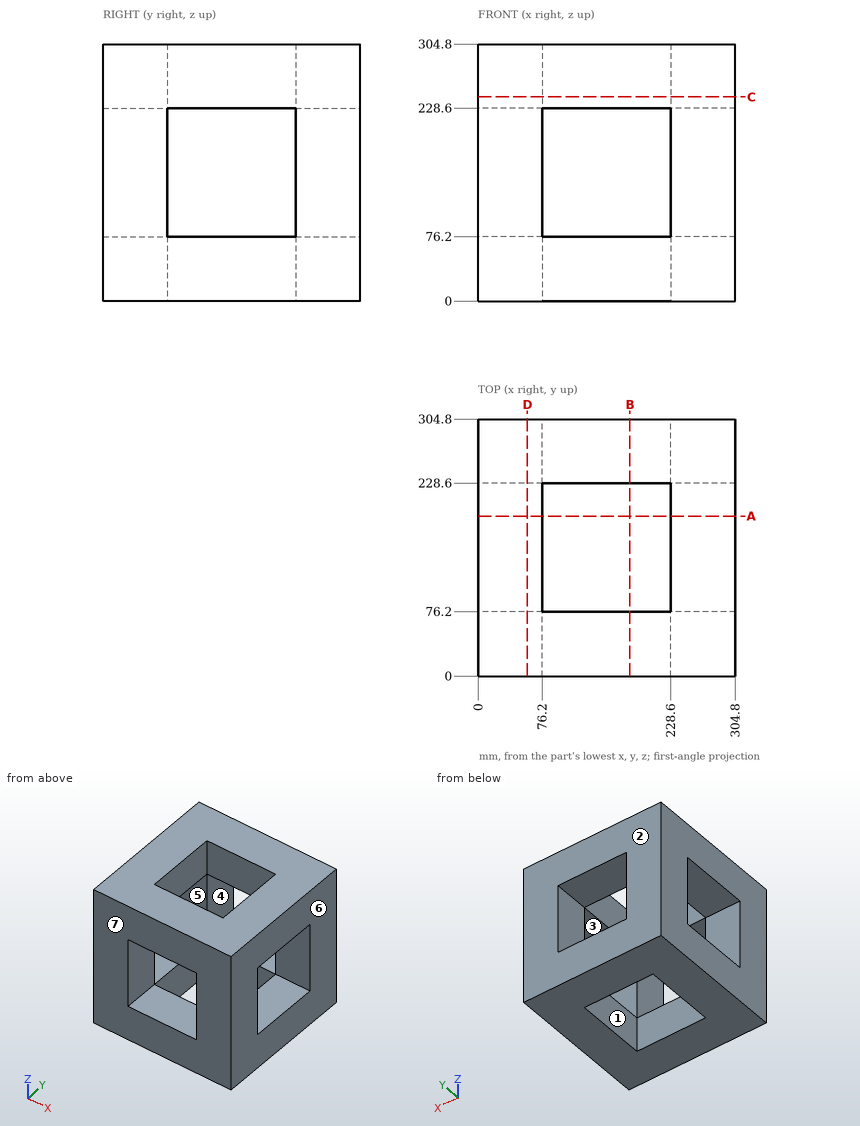
Print and shaded views of the part. All mm, measured from the part's lowest x, y and z. A direction names the side the tool comes from. Coordinates: 2 decimals unless noted, no trailing zeros. Order: outer loops, then holes, each group sorted by start corner. A loop starts at its lowest first (then second) coordinate and runs counter-clockwise, first axis right, second up. Notation, with made-up numbers: (54.25, -39.75) -> (99.25, -39.75) arc R18 cw to (99.25, -8.75) -> close; hole circle Ø2 at (4, 1). An arc over 180 degrees is marked (long way). Answer as a JSON object with one key per item and string values. Group by question number.
1) Cut at A-A, the plane y = 189.5. Write the cut outline in (x, z), then the cut area to 3 significant figures.
2) Which spindle directions (+Z, -Z, +X, -X, +Y, -Y) get a long thin tool onto all of the face, cutting with end or side? Do the marked faces 1, 2, 3 and 4. Say none if no direction does.
3) Pull direction Y, two halves, no side cores. Call the marked faces 5, 6 and 7: +Y half, -Y half, draft (parallel to the pull), parting line (faces both ways), or undercut.
4) Drill centre line: L1, parallel to Y at x = 220, z = 72. Where is it in solid material? Low to high.
5) Flat gauge pin, fed straight in: pin 1 (23 mm diameter, centred on x = 143, y = 50, fed in from -Z). Where does the tip first touch, or does it go through?
6) Cut at C-C, the plane z = 242. Write the cut outline in (x, y), then the cut area to 3 significant figures.
Check values:
{
 "1": {"outline": "(0, 0) -> (76.2, 0) -> (76.2, 76.2) -> (0, 76.2) -> close; (0, 228.6) -> (76.2, 228.6) -> (76.2, 304.8) -> (0, 304.8) -> close; (228.6, 0) -> (304.8, 0) -> (304.8, 76.2) -> (228.6, 76.2) -> close; (228.6, 228.6) -> (304.8, 228.6) -> (304.8, 304.8) -> (228.6, 304.8) -> close", "area": "23,200 mm²"},
 "2": {"face 1": "+Z, -Z", "face 2": "+Z, -Z, +X, -X, +Y", "face 3": "+X, -X", "face 4": "+Y, -Y"},
 "3": {"face 5": "undercut", "face 6": "draft", "face 7": "-Y half"},
 "4": {"L1": "y = 0 to 76.2, 228.6 to 304.8"},
 "5": {"pin 1": "stops at z = 0"},
 "6": {"outline": "(0, 0) -> (304.8, 0) -> (304.8, 304.8) -> (0, 304.8) -> close; hole (76.2, 76.2) -> (228.6, 76.2) -> (228.6, 228.6) -> (76.2, 228.6) -> close", "area": "69,700 mm²"}
}
